Model file for the job. Use its own axes, mm. A direction names the side the tool comes from. Give positions to 0.01 mm unless a question says otherwise; leave off trailing zeros. Loops run counter-clockwise (first coordinate to the right, second up) from the corner with the lowest first, then second, coordinate; pieces in that order, holes last. Notation, with made-up numbers: (43, 0.25) - (49, 0.25) arc R19 ccw to (49, 31.25) - close; hole circle Ø3 at (80, -5.75). An arc over 180 degrees is marked (long way). Use a Markdown table: item, result.
from build123d import *

# Parameters (mm, degrees)
SKETCH_1_W          = 15
SKETCH_1_H          = 15
SKETCH_1_W_2        = 13
SKETCH_1_H_2        = 13
EXTRUDE_1_DEPTH     = 570
SKETCH_2_R          = 1.45
CUT_EXTRUDE_1_DEPTH = 571.246657158
SKETCH_3_R          = 1.45
CUT_EXTRUDE_2_DEPTH = 571.246657158


with BuildPart() as part:
    # 草图1 → 凸台-拉伸1 (new body)
    with BuildSketch(Plane(origin=(0, 0, 0), x_dir=(0, 0, -1), z_dir=(1, 0, 0))):
        Rectangle(SKETCH_1_W, SKETCH_1_H)
        Rectangle(SKETCH_1_W_2, SKETCH_1_H_2, mode=Mode.SUBTRACT)
    extrude(amount=EXTRUDE_1_DEPTH)

    # 草图2 → 切除-拉伸1 (cut, through all)
    with BuildSketch(Plane(origin=(0, 7.5, 0), x_dir=(1, 0, 0), z_dir=(0, 1, 0))):
        with Locations(Location((560.5, 0, 0), (0, 0, 270))):
            Circle(SKETCH_2_R)
        with Locations(Location((547, 0, 0), (0, 0, 270))):
            Circle(SKETCH_2_R)
        with Locations(Location((399, 0, 0), (0, 0, 270))):
            Circle(SKETCH_2_R)
        with Locations(Location((356, 0, 0), (0, 0, 270))):
            Circle(SKETCH_2_R)
        with Locations(Location((214, 0, 0), (0, 0, 270))):
            Circle(SKETCH_2_R)
        with Locations(Location((171, 0, 0), (0, 0, 270))):
            Circle(SKETCH_2_R)
        with Locations(Location((23, 0, 0), (0, 0, 270))):
            Circle(SKETCH_2_R)
        with Locations(Location((9.5, 0, 0), (0, 0, 270))):
            Circle(SKETCH_2_R)
        with Locations(Location((472.5, 0, 0), (0, 0, 270))):
            Circle(SKETCH_2_R)
        with Locations(Location((57.5, 0, 0), (0, 0, 270))):
            Circle(SKETCH_2_R)
        with Locations(Location((77.5, 0, 0), (0, 0, 270))):
            Circle(SKETCH_2_R)
        with Locations(Location((492.5, 0, 0), (0, 0, 270))):
            Circle(SKETCH_2_R)
        with Locations(Location((512.5, 0, 0), (0, 0, 270))):
            Circle(SKETCH_2_R)
        with Locations(Location((272.5, 0, 0), (0, 0, 270))):
            Circle(SKETCH_2_R)
        with Locations(Location((297.5, 0, 0), (0, 0, 270))):
            Circle(SKETCH_2_R)
        with Locations(Location((97.5, 0, 0), (0, 0, 270))):
            Circle(SKETCH_2_R)
    extrude(amount=-CUT_EXTRUDE_1_DEPTH, mode=Mode.SUBTRACT)

    # 草图3 → 切除-拉伸2 (cut, through all)
    with BuildSketch(Plane(origin=(0, 0, -7.5), x_dir=(-1, 0, 0), z_dir=(0, 0, -1))):
        with Locations((-176, 0)):
            Circle(SKETCH_3_R)
        with Locations((-209, 0)):
            Circle(SKETCH_3_R)
        with Locations((-361, 0)):
            Circle(SKETCH_3_R)
        with Locations((-394, 0)):
            Circle(SKETCH_3_R)
    extrude(amount=-CUT_EXTRUDE_2_DEPTH, mode=Mode.SUBTRACT)


solid = part.part
(1) Pin check, flat tip, straight feed: P1, Ø2.5, axis at x = 547, z = 0, coming from the +Y side. Stop position of the tip, or through.
Computed:
| item | result |
|---|---|
| P1 | through |
(2) Mould opens along Z. For faces 3 (the flat face through (0, 0, 7)), 4 (the flat face through (281, 0, -6.5)), 5 (the flat face through (281, -6.5, 0)), 6 (the flat face through (281, 0, -7.5)) say: pulls with the +Z half, pulls with the -Z half, needs draft (parallel to the pull), parting line crosses it, or undercut.
Computed:
| item | result |
|---|---|
| face 3 | needs draft |
| face 4 | undercut |
| face 5 | undercut |
| face 6 | pulls with the -Z half |
(3) Slice it at A-A, the plane x = 128.5. Write the cut outline in (y, z).
Computed:
| item | result |
|---|---|
| outline | (-7.5, -7.5) - (7.5, -7.5) - (7.5, 7.5) - (-7.5, 7.5) - close; hole (-6.5, -6.5) - (6.5, -6.5) - (6.5, 6.5) - (-6.5, 6.5) - close |
(4) 3-axis set-ups, long thin cutter, end or side, ignore diameter. For faces 1 (the flat face through (281, 6.5, 0)), 2 (the flat face through (281, 0, 7.5)): which of +Z, -Z, +X, -X, +Y, -Y reach the whole face in a straight line?
Computed:
| item | result |
|---|---|
| face 1 | +X, -X |
| face 2 | +Z, +X, -X, +Y, -Y |
(5) Drill centre lines: probe 1 along Z at (x, y) = (272.5, -6.9); probe 2 along Y at (x, z) = (335, 0.25). Where is each one in solid material? Low to high. Write a range as [from, to].
Computed:
| item | result |
|---|---|
| probe 1 | [-7.5, -1.45], [1.45, 7.5] |
| probe 2 | [-7.5, -6.5], [6.5, 7.5] |
